Check sheet for the modelled part. Datum: model origin and axes. Units: mm. Give positions to 0.01 mm unless a question says otherwise; leave off trailing zeros. Write each loop counter-clockwise with the first axis right and the second up, starting at its lowest first coordinate (ties: lowest second). Pieces come first, ordered by that corner, then holes.
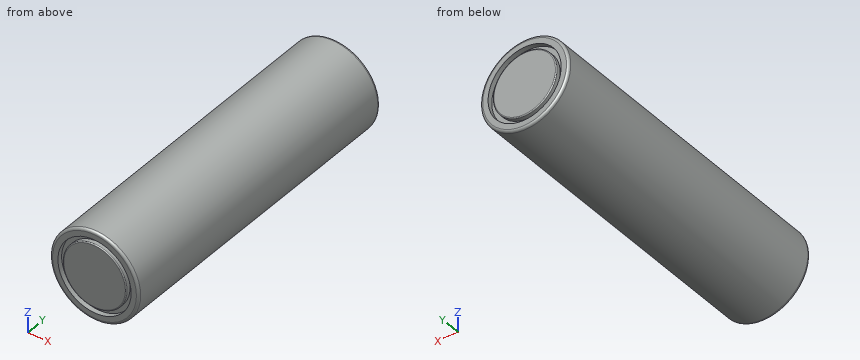
from build123d import *

# Parameters (mm, degrees)
SKETCH1_R           = 9.1
BOSS_EXTRUDE1_DEPTH = 65
SKETCH2_R           = 7.515816548
SKETCH2_R_2         = 6.528062022
CUT_EXTRUDE1_DEPTH  = 1
FILLET1_R           = 0.5
SKETCH3_R           = 7.515816548
SKETCH3_R_2         = 6.528062022
CUT_EXTRUDE2_DEPTH  = 1
FILLET2_R           = 0.2


with BuildPart() as part:
    # Sketch1 → Boss-Extrude1 (new body)
    with BuildSketch(Plane(origin=(0, 0, 0), x_dir=(1, 0, 0), z_dir=(0, 1, 0))):
        Circle(SKETCH1_R)
    extrude(amount=BOSS_EXTRUDE1_DEPTH)

    # Sketch2 → Cut-Extrude1 (cut)
    with BuildSketch(Plane(origin=(0, 65, 0), x_dir=(1, 0, 0), z_dir=(0, 1, 0))):
        Circle(SKETCH2_R)
        Circle(SKETCH2_R_2, mode=Mode.SUBTRACT)
    extrude(amount=-CUT_EXTRUDE1_DEPTH, mode=Mode.SUBTRACT)

    # Fillet1
    fillet1_edges = [part.edges().sort_by_distance(p)[0] for p in [
        (-9.1, 0, 0),
        (-9.1, 65, 0),
    ]]
    fillet(fillet1_edges, radius=FILLET1_R)

    # Sketch3 → Cut-Extrude2 (cut)
    with BuildSketch(Plane.XZ):
        Circle(SKETCH3_R)
        Circle(SKETCH3_R_2, mode=Mode.SUBTRACT)
    extrude(amount=-CUT_EXTRUDE2_DEPTH, mode=Mode.SUBTRACT)

    # Fillet2
    fillet2_edges = [part.edges().sort_by_distance(p)[0] for p in [
        (-6.528062022, 0, 0),
        (-6.528062022, 65, 0),
    ]]
    fillet(fillet2_edges, radius=FILLET2_R)


solid = part.part
1) Gauge pin test, flat ends, axial feed: pin 1 (3 mm diameter, centred on x = 4.5, y = 20, fed in from -Z); pin 2 (10 mm diameter, centred on y = 32, z = 7, fed in from +X); pin 3 (2 mm diameter, centred on x = 2.5, y = 48.5, fed in from +Z). Record the tip position at first contact, or that the pin passes through.
2) Scan lines: L1, parallel to Z at x = 0, y = 64.6; L2, parallel to X at y = 64.3, z = 0; L3, parallel to Z at x = 0, y = 0.25. Record each from-to range of solid material in increasing order.
3) Sectioned sample at A-A on y = 48. Record the boundary of the cut face in (x, z).
Answers below:
1. pin 1: stops at z = -8.59
1. pin 2: stops at x = 8.88
1. pin 3: stops at z = 8.98
2. L1: z = -9.09 to -7.52, -6.53 to 6.53, 7.52 to 9.09
2. L2: x = -9.1 to -7.52, -6.53 to 6.53, 7.52 to 9.1
2. L3: z = -9.03 to -7.52, -6.53 to 6.53, 7.52 to 9.03
3. outline: circle Ø18.2 at (0, 0)
